The model under review builds one solid part; all positions refer to its coordinate system, in mm. Give positions to 0.01 mm unless a question says otherwise; leave off trailing zeros. Order: outer loops, then holes, each group sorted by start corner. A loop starts at its lowest first (then second) coordinate and runs counter-clockwise, first axis right, second up. Notation, with made-up numbers: (50, 20) - (102, 20) arc R18 ccw to (102, 55) - close; hole circle Ø5 at (33, 82). An arc over 180 degrees is marked (long way). Use a Markdown table: item, result. Add a question column.
Solid Edge part; units mm, degrees
sketch "Sketch1" plane through (0, 0, 0) normal (0, 0, 1) x (1, 0, 0)
  line L0 (10, -17.3205) -> (20, 0)
  line L1 (20, 0) -> (10, 17.3205)
  line L2 (10, 17.3205) -> (-10, 17.3205)
  line L3 (-10, 17.3205) -> (-20, 0)
  line L4 (-10, -17.3205) -> (-20, 0)
  line L5 (10, -17.3205) -> (-10, -17.3205)
extrude "Protrusion1" add sketch "Sketch1" along normal mid plane 16
hole "Hole_1" at (0, 0, 8) direction (0, 0, -1) diameter 17.294 end through all
sketch "Sketch2" plane through (0, 0, 0) normal (1, 0, 0) x (0, 1, 0)
  line L0 (17.3205, -8) -> (33.7074, 1.461)
revolve "RevolvedCutout1" cut sketch "Sketch2" angle 360 about axis through (0, 0, -57) along (0, 0, 1) material side at (0, 25.539, -3.3128)
mirror "Mirror1" about plane through (0, 0, 0) normal (0, 0, 1) of "RevolvedCutout1"
properties part number "6" material "Fe 410 W"
Q1. We need section A-A (z = -5). Write out the cut boundary in (x, y), plus the area to 3 significant figures.
Q2. Clearance check with flat-ended pins moving along their axes: P1, Ø6, axis at x = -13, y = 13, coming from the +Z side; P2, Ø1, axis at x = 12.5, z = 0.5, coming from the -Y side. State where each tip first meets the part, or that it passes through.
Q3. Wall thickness on probe 1 along X at (y, z) = (0, 0.75); probe 2 along Y at (x, z) = (0, 0.5); probe 3 along Y at (x, z) = (-6.5, 2.75): over which ranges is each line inside the solid? List them lowest first.
Here are the results:
| question | item | result |
|---|---|---|
| 1 | outline | (-20, 0) - (-10, -17.32) - (10, -17.32) - (20, 0) - (10, 17.32) - (-10, 17.32) - close; hole circle Ø17.29 at (0, 0) |
| 1 | area | 804 mm2 |
| 2 | P1 | z = 8 |
| 2 | P2 | y = -13.86 |
| 3 | probe 1 | -20 to -8.65, 8.65 to 20 |
| 3 | probe 2 | -17.32 to -8.65, 8.65 to 17.32 |
| 3 | probe 3 | -17.32 to -5.7, 5.7 to 17.32 |
